The listing builds one solid part. Answer for the finished solid, in the listing's coordinates (mm). A direction names the side the tool comes from. Give positions to 0.01 mm unless a question says otherwise; leave off trailing zeros. Order: outer loops, then holes, each group sorted by start corner. A loop starts at its lowest first (then second) coordinate and runs counter-clockwise, first axis right, second up. Notation, with made-up numbers: (63, 22) - (86, 22) arc R27 cw to (86, 38) - close; hole circle Ø6 at (73.25, 34). An arc over 180 degrees is marked (long way). Answer as CSV lines item,"result". Start each with the question number.
1. Flat-ended cylindrical pins translate along their axes: pin 1 (4.5 mm diameter, centred on x = -22.5, y = 31, fed in from +Z); pin 2 (6 mm diameter, centred on x = 13.5, y = 22.5, fed in from +Z) (3 decimals); pin 3 (2.5 mm diameter, centred on y = 36, z = -24, fed in from -X). Find the tip coordinate at first contact, or state that the pin passes through.
2. Section B-B on y = 28 is taken. Give the vertices of the cut face in (x, z) (3 decimals).
3. Section C-C on z = 0 is taken. Give the vertices of the cut face in (x, y) (3 decimals).
4. Consider line 1 along Z through (x, y) = (0, 1.25) (3 decimals); line 2 along Y through (x, z) = (-1, 12); line 3 along Y through (x, z) = (16, 16). Determine where each line is inside the solid, lowest interval first. Write a range as [from, to].
5. Section D-D on z = 7.5 is taken. Give the vertices of the cut face in (x, y) (3 decimals).
6. Section A-A on x = 0 is taken. Give the vertices of the cut face in (y, z) (3 decimals), and give its area (3 significant figures).
7. Which of the six approach directions +Z, -Z, +X, -X, +Y, -Y give full straight-line access (tool end or side, diameter ignored) to faces 1 (the flat face through (24, 25, 19.5)), 2 (the cylindrical face through (-0.59, 1.16, 4.46)), 3 (the flat face through (-24, 27, 19.5)), 4 (the flat face through (10.5, 6, 33))?
8. Determine the mould class of faces 5 (the flat face through (0, 2.35, 0)), 6 (the cylindrical face through (8.767, 56.109, 16.856)), 7 (the flat face through (-19.5, 27, 24)) for opening direction Z: +Z half, -Z half, draft (parallel to the pull), parting line (faces both ways), or undercut.
from build123d import *

# Parameters (mm, degrees)
SKETCH1_W           = 56.45
SKETCH1_H           = 56.45
BOSS_EXTRUDE1_DEPTH = 55
SKETCH2_R           = 19
BOSS_EXTRUDE2_DEPTH = 2.25
SKETCH3_R           = 3.2
BOSS_EXTRUDE3_DEPTH = 30
SKETCH4_W           = 8.725
SKETCH4_H           = 8.725
CUT_EXTRUDE1_DEPTH  = 55
SKETCH4_3_W         = 8.725
SKETCH4_3_H         = 8.725
CUT_EXTRUDE2_DEPTH  = 50
BOSS_EXTRUDE4_DEPTH = 11.6
SKETCH6_R           = 2.5
CUT_EXTRUDE3_DEPTH  = 5
SKETCH7_R           = 4.5
CUT_EXTRUDE4_DEPTH  = 2.35


with BuildPart() as part:
    # Sketch1 → Boss-Extrude1 (new body)
    with BuildSketch(Plane(origin=(0, 0, 0), x_dir=(1, 0, 0), z_dir=(0, 1, 0))):
        Rectangle(SKETCH1_W, SKETCH1_H)
    extrude(amount=BOSS_EXTRUDE1_DEPTH)

    # Sketch2 → Boss-Extrude2 (add)
    with BuildSketch(Plane(origin=(0, 55, 0), x_dir=(1, 0, 0), z_dir=(0, 1, 0))):
        Circle(SKETCH2_R)
    extrude(amount=BOSS_EXTRUDE2_DEPTH)

    # Sketch3 → Boss-Extrude3 (add)
    with BuildSketch(Plane(origin=(0, 57.25, 0), x_dir=(1, 0, 0), z_dir=(0, 1, 0))):
        Circle(SKETCH3_R)
    extrude(amount=BOSS_EXTRUDE3_DEPTH)

    # Sketch4 → Cut-Extrude1 (cut)
    with BuildSketch(Plane.XZ):
        with Locations((23.8625, -23.8625)):
            Rectangle(SKETCH4_W, SKETCH4_H)
        with Locations((-23.8625, 23.8625)):
            Rectangle(SKETCH4_W, SKETCH4_H)
    extrude(amount=-CUT_EXTRUDE1_DEPTH, mode=Mode.SUBTRACT)

    # Sketch4<3> → Cut-Extrude2 (cut)
    with BuildSketch(Plane.XZ):
        with Locations((23.8625, 23.8625)):
            Rectangle(SKETCH4_3_W, SKETCH4_3_H)
        with Locations((-23.8625, -23.8625)):
            Rectangle(SKETCH4_3_W, SKETCH4_3_H)
    extrude(amount=-CUT_EXTRUDE2_DEPTH, mode=Mode.SUBTRACT)

    # Sketch5 → Boss-Extrude4 (add)
    with BuildSketch(Plane.XZ):
        Polygon((0, 28.225), (10.5, 28.225), (10.5, 38.225), (-10.5, 38.225), (-10.5, 28.225), align=None)
    extrude(amount=-BOSS_EXTRUDE4_DEPTH)

    # Sketch6 → Cut-Extrude3 (cut)
    with BuildSketch(Plane(origin=(0, 55, 0), x_dir=(1, 0, 0), z_dir=(0, 1, 0))):
        with Locations((-23.175, 23.175)):
            Circle(SKETCH6_R)
        with Locations((23.175, -23.175)):
            Circle(SKETCH6_R)
    extrude(amount=-CUT_EXTRUDE3_DEPTH, mode=Mode.SUBTRACT)

    # Sketch7 → Cut-Extrude4 (cut)
    with BuildSketch(Plane.XZ):
        Circle(SKETCH7_R)
    extrude(amount=-CUT_EXTRUDE4_DEPTH, mode=Mode.SUBTRACT)


solid = part.part
Checks:
1,pin 1,"stops at z = 19.5"
1,pin 2,"stops at z = 28.225"
1,pin 3,"stops at x = -19.5"
2,outline,"(-28.225, -19.5) - (-19.5, -19.5) - (-19.5, -28.225) - (19.5, -28.225) - (19.5, -19.5) - (28.225, -19.5) - (28.225, 19.5) - (19.5, 19.5) - (19.5, 28.225) - (-19.5, 28.225) - (-19.5, 19.5) - (-28.225, 19.5) - close"
3,outline,"(-28.225, 0) - (-4.5, 0) - (-4.5, 2.35) - (4.5, 2.35) - (4.5, 0) - (28.225, 0) - (28.225, 55) - (19, 55) - (19, 57.25) - (3.2, 57.25) - (3.2, 87.25) - (-3.2, 87.25) - (-3.2, 57.25) - (-19, 57.25) - (-19, 55) - (-28.225, 55) - close"
4,line 1,"z = [-28.225, -4.5], [4.5, 38.225]"
4,line 2,"y = [0, 57.25]"
4,line 3,"y = [0, 55]"
5,outline,"(-28.225, 0) - (28.225, 0) - (28.225, 55) - (17.457, 55) - (17.457, 57.25) - (-17.457, 57.25) - (-17.457, 55) - (-28.225, 55) - close"
6,outline,"(0, -28.225) - (55, -28.225) - (55, -19) - (57.25, -19) - (57.25, -3.2) - (87.25, -3.2) - (87.25, 3.2) - (57.25, 3.2) - (57.25, 19) - (55, 19) - (55, 28.225) - (11.6, 28.225) - (11.6, 38.225) - (0, 38.225) - (0, 4.5) - (2.35, 4.5) - (2.35, -4.5) - (0, -4.5) - close"
6,area,"3,480 mm²"
7,face 1,"+Z, +X, -Y"
7,face 2,"-Y"
7,face 3,"+Z, -X, +Y, -Y"
7,face 4,"+Z, +X, +Y, -Y"
8,face 5,"undercut"
8,face 6,"parting line"
8,face 7,"draft"
